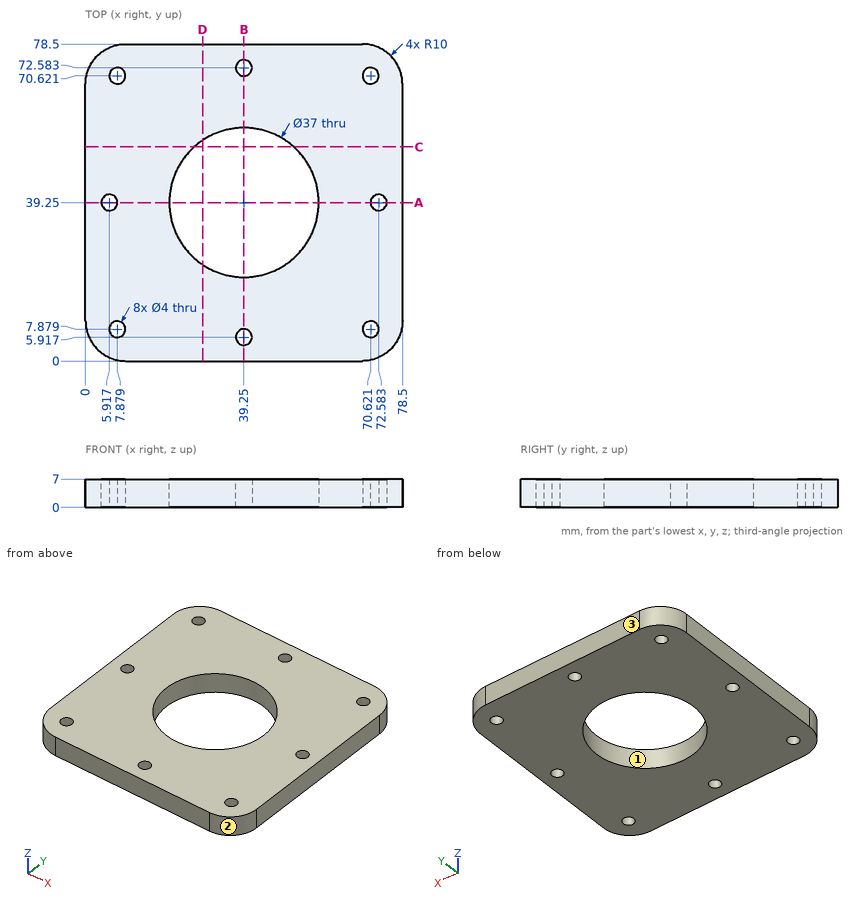
Verification items for this drawing (mm, ordinates from the low corner). Round coordinates to 2 decimals unless told otherwise and drop trailing zeros. Order: outer loops, then holes, each group sorted by start corner. A loop starts at its lowest first (then second) coordinate and runs counter-clockwise, first axis right, second up. Notation, with made-up numbers: (-27, 22.25) - (23, 22.25) arc R25 ccw to (23, 50.25) - close; hole circle Ø2 at (-17, 4). An arc over 180 degrees is marked (long way). Answer as CSV lines item,"result". Start each with the question number.
1) Section check C-C (y = 53). Record the cut outline in (x, z).
2) Section check D-D (x = 29). Record the cut outline in (y, z).
3) Draft check along X on the marked faces 1, 2 and 3. Enter one of: +X half, -X half, draft (parallel to the pull), parting line (faces both ways), or undercut.
4) Scan lines: probe 1 along Y at (x, z) = (39.25, 2.5); probe 2 along Y at (x, z) = (6.5, 1.75) (1 decimal); probe 3 along X at (y, z) = (47, 3.5). Record each from-to range of solid material in increasing order.
5) Depth check by flat-ended pin: pin 1 (5 mm diameter, centred on x = 48, y = 50.5, fed in from -Z). Enter the tip coordinate at first touch or a pass-through.
6) Section check A-A (y = 39.25). Record the cut outline in (x, z).
Determined:
1,outline,"(0, 0) - (26.87, 0) - (26.87, 7) - (0, 7) - close; (51.63, 0) - (78.5, 0) - (78.5, 7) - (51.63, 7) - close"
2,outline,"(0, 0) - (23.85, 0) - (23.85, 7) - (0, 7) - close; (54.65, 0) - (78.5, 0) - (78.5, 7) - (54.65, 7) - close"
3,face 1,"undercut"
3,face 2,"+X half"
3,face 3,"draft"
4,probe 1,"0 to 3.92, 7.92 to 20.75, 57.75 to 70.58, 74.58 to 78.5"
4,probe 2,"0.6 to 6.4, 9.3 to 37.3, 41.2 to 69.2, 72.1 to 77.9"
4,probe 3,"0 to 22.45, 56.05 to 78.5"
5,pin 1,"through"
6,outline,"(0, 0) - (3.92, 0) - (3.92, 7) - (0, 7) - close; (7.92, 0) - (20.75, 0) - (20.75, 7) - (7.92, 7) - close; (57.75, 0) - (70.58, 0) - (70.58, 7) - (57.75, 7) - close; (74.58, 0) - (78.5, 0) - (78.5, 7) - (74.58, 7) - close"
